Read the model definition and answer for the solid it produces. Units are mm, in the model's axes. A direction names the side the tool comes from. Give positions to 0.01 mm unless a question says otherwise; leave off trailing zeros. Answer as CSV lines item,"result". Start each with the question number.
```python
from build123d import *

# Parameters (mm, degrees)
REVOLVE_1_ANGLE          = 40
SKETCH_4_W               = 4.8
SKETCH_4_H               = 4.8
EXTRUDE_1_DEPTH          = 6
SKETCH_7_R               = 1.5
CUT_EXTRUDE_4_DEPTH      = 95.895882206
SKETCH_13_R              = 1.5
CUT_EXTRUDE_7_DEPTH      = 57.80711304
CUT_EXTRUDE_8_DEPTH      = 5
SKETCH_16_W              = 3
SKETCH_16_H              = 3
PATTERN_CIRCULAR_1_COUNT = 4
PATTERN_CIRCULAR_1_ANGLE = 15
SKETCH_10_W              = 2.2
SKETCH_10_H              = 5.2
CUT_EXTRUDE_5_DEPTH      = 3
SKETCH_11_W              = 47.375376564
SKETCH_11_H              = 32.407082742
CUT_EXTRUDE_6_DEPTH      = 149.607349927
SKETCH_12_W              = 14
SKETCH_12_H              = 30
EXTRUDE_2_DEPTH          = 5
FILLET_1_R               = 5


# Read off the part's stored shape, not the designer's step: 旋转1
with BuildPart() as part:
    # 旋转1 outline → 旋转1 (revolve)
    with BuildSketch(Plane(origin=(0, 0, 0), x_dir=(0.3420201433256701, 0, -0.9396926207859079), z_dir=(0.9396926207859079, 0, 0.3420201433256701))):
        Polygon((134, 5), (125, 5), (125, -5), (134, -5), (134, -7.5), (136.5, -10), (139, -7.5), (139, 7.5), (136.5, 10), (134, 7.5), align=None)
    revolve(axis=Axis((0, 0, 0), (0, 1, 0)), revolution_arc=REVOLVE_1_ANGLE)

    # 草图4 → 凸台-拉伸1 (add)
    with BuildSketch(Plane(origin=(0, 0, 0), x_dir=(0.3420201433256631, 0, 0.9396926207859104), z_dir=(-0.9396926207859104, 0, 0.3420201433256631))):
        with Locations((-132, 0)):
            Rectangle(SKETCH_4_W, SKETCH_4_H)
    extrude(amount=EXTRUDE_1_DEPTH)

    # 草图7 → 切除-拉伸4 (cut, through all)
    with BuildSketch(Plane(origin=(-45.967507263, 0, -126.294688234), x_dir=(-0.9396926207859105, 0, 0.3420201433256632), z_dir=(-0.3420201433256632, 0, -0.9396926207859105))):
        with Locations((3, 0)):
            Circle(SKETCH_7_R)
    extrude(amount=-CUT_EXTRUDE_4_DEPTH, mode=Mode.SUBTRACT)

    # 草图13 → 切除-拉伸7 (cut, through all)
    with BuildSketch(Plane(origin=(0, 0, -139), x_dir=(-1, 0, 0), z_dir=(0, 0, -1))):
        Circle(SKETCH_13_R)
    cut_extrude_7 = extrude(amount=-CUT_EXTRUDE_7_DEPTH, mode=Mode.SUBTRACT)

    # 草图14 → 切除-拉伸8 (cut)
    with BuildSketch(Plane(origin=(0, 0, -139), x_dir=(-1, 0, 0), z_dir=(0, 0, -1))):
        Polygon((0, -3.175426481), (2.75, -1.58771324), (2.75, 1.58771324), (0, 3.175426481), (-2.75, 1.58771324), (-2.75, -1.58771324), align=None)
    cut_extrude_8 = extrude(amount=-CUT_EXTRUDE_8_DEPTH, mode=Mode.SUBTRACT)

    # 草图16 → 切除-旋转1 (revolve, cut)
    with BuildSketch(Plane(origin=(0, 0, 0), x_dir=(1, 0, 0), z_dir=(0, 1, 0)), mode=Mode.PRIVATE) as cut_revolve_1_sk:
        with Locations((1.5, 126.463994814)):
            Rectangle(SKETCH_16_W, SKETCH_16_H)
    cut_revolve_1 = revolve(cut_revolve_1_sk.sketch.rotate(Axis((0, 0, 999.226836895), (0, 0, -1)), 180), axis=Axis((0, 0, 999.226836895), (0, 0, -1)), mode=Mode.SUBTRACT)

    # 阵列(圆周)1: 切除-拉伸7, 切除-拉伸8, 切除-旋转1 ×4 about axis
    pattern_circular_1_axis = Axis((0, 0, 0), (0, 1, 0))
    add([cut_extrude_7.rotate(pattern_circular_1_axis, i * PATTERN_CIRCULAR_1_ANGLE / (PATTERN_CIRCULAR_1_COUNT - 1)) for i in range(1, PATTERN_CIRCULAR_1_COUNT)], mode=Mode.SUBTRACT)
    add([cut_extrude_8.rotate(pattern_circular_1_axis, i * PATTERN_CIRCULAR_1_ANGLE / (PATTERN_CIRCULAR_1_COUNT - 1)) for i in range(1, PATTERN_CIRCULAR_1_COUNT)], mode=Mode.SUBTRACT)
    add([cut_revolve_1.rotate(pattern_circular_1_axis, i * PATTERN_CIRCULAR_1_ANGLE / (PATTERN_CIRCULAR_1_COUNT - 1)) for i in range(1, PATTERN_CIRCULAR_1_COUNT)], mode=Mode.SUBTRACT)

    # 草图10 → 切除-拉伸5 (cut)
    with BuildSketch(Plane(origin=(0, 0, 0), x_dir=(0.3420201433256631, 0, 0.9396926207859104), z_dir=(-0.9396926207859104, 0, 0.3420201433256631))):
        with Locations((-137.9, 0)):
            Rectangle(SKETCH_10_W, SKETCH_10_H)
        Polygon((-127.2, 5), (-125, 5), (-123.655375964, 5), (-123.655375964, 1.8), (-125, 1.8), (-127.2, 1.8), align=None)
        Polygon((-127.2, -1.8), (-125, -1.8), (-123.655375964, -1.8), (-123.655375964, -5), (-125, -5), (-127.2, -5), align=None)
    extrude(amount=-CUT_EXTRUDE_5_DEPTH, mode=Mode.SUBTRACT)

    # 草图11 → 切除-拉伸6 (cut, through all)
    with BuildSketch(Plane(origin=(0, 0, 0), x_dir=(0, -1, 0), z_dir=(0.9990482215818578, 0, 0.0436193873653361))):
        with Locations((-1.017262687, 125.577370773)):
            Rectangle(SKETCH_11_W, SKETCH_11_H)
    extrude(amount=CUT_EXTRUDE_6_DEPTH, mode=Mode.SUBTRACT)

    # 草图12 → 凸台-拉伸2 (add)
    with BuildSketch(Plane(origin=(0, 0, 0), x_dir=(0.043619387365336125, 0, -0.9990482215818578), z_dir=(0.9990482215818577, 0, 0.04361938736533612))):
        with Locations((132, 0)):
            Rectangle(SKETCH_12_W, SKETCH_12_H)
    extrude(amount=EXTRUDE_2_DEPTH)

    # 圆角1
    fillet_1_edges = [part.edges().sort_by_distance(p)[0] for p in [
        (7.950043975, 15, -124.771979229),
        (7.950043975, -15, -124.771979229),
        (8.560715398, -15, -138.758654331),
        (8.560715398, 15, -138.758654331),
    ]]
    fillet(fillet_1_edges, radius=FILLET_1_R)


solid = part.part
```
1. Find the intervals of material crossed by line 1 (Y direction, x = 0, z = -129.5); line 2 (Y direction, x = -41, z = -126); line 3 (Y direction, x = 0, z = -126.2), in increasing order. Write a range as [from, to].
2. Find section A-A on y = 0. State how many separate pieces and enclosed holes the cut face has, then the cut area to 3 significant figures.
3. Given pin 1 (3.5 mm diameter, centred on x = -49, z = -124, fed in from -Y); pin 2 (2.5 mm diameter, centred on x = -42, z = -119.5, fed in from -Y); pin 3 (2.5 mm diameter, centred on x = -45, z = -130, fed in from -Y); pin 4 (2.5 mm diameter, centred on x = 0, y = 0, fed in from -Z), each flat-ended and moving along its own axis, determine where each tip first touches the part or whether it passes through.
4. For faces 1 (the face through (1.5, 0.07, -131.02)), 2 (the face through (1.36, 2.39, -136.54)), 3 (the face through (-9.16, 0.02, -136.24)), 4 (the face through (-2.86, 0.9, -126.48)), 5 (the face through (10.75, 0.21, -131.56)), determine the directions among +Z, -Z, +X, -X, +Y, -Y from which every point of the face is accessible in a straight line to the end or side of a thin tool.
5. Determine the mould class of faces 6 (the face through (1.3, -1.4, -134)), 7 (the face through (-42, -1.8, -119)), 8 (the face through (-20.998, 0.022, -134.925)) for opening direction Z: +Z half, -Z half, draft (parallel to the pull), parting line (faces both ways), or undercut.
Computed:
1,line 1,"y = [-5, -1.5], [1.5, 5]"
1,line 2,"y = [-5, 5]"
1,line 3,"y = [-5, -3], [3, 5]"
2,separate pieces,"6"
2,enclosed holes,"0"
2,area,"550 mm^2"
3,pin 1,"stops at y = -2.4"
3,pin 2,"stops at y = -5"
3,pin 3,"stops at y = -10"
3,pin 4,"passes through"
4,face 1,"+Z, -Z"
4,face 2,"-Z"
4,face 3,"none"
4,face 4,"+Z"
4,face 5,"+Z, +X, +Y, -Y"
5,face 6,"-Z half"
5,face 7,"draft"
5,face 8,"undercut"
